```python
from build123d import *

# Parameters (mm, degrees)
SKETCH1_W           = 200
SKETCH1_H           = 200.3
BOSS_EXTRUDE1_DEPTH = 18
FILLET1_R           = 10
SKETCH2_W           = 150
SKETCH2_H           = 100
CUT_EXTRUDE1_DEPTH  = 13
FILLET2_R           = 10
SKETCH3_R           = 5
CUT_EXTRUDE2_DEPTH  = 5
SKETCH4_R           = 2.5
CUT_EXTRUDE3_DEPTH  = 143.123265161
SKETCH5_R           = 10
CUT_EXTRUDE4_DEPTH  = 143.123265161
SKETCH6_R           = 1.5
SKETCH6_W           = 23
SKETCH6_H           = 10
CUT_EXTRUDE5_DEPTH  = 143.667524335
FILLET3_R           = 3


with BuildPart() as part:
    # Sketch1 → Boss-Extrude1 (new body)
    with BuildSketch(Plane(origin=(0, 0, 0), x_dir=(1, 0, 0), z_dir=(0, 1, 0))):
        Rectangle(SKETCH1_W, SKETCH1_H)
    extrude(amount=BOSS_EXTRUDE1_DEPTH)

    # Fillet1
    fillet1_edges = [part.edges().sort_by_distance(p)[0] for p in [
        (100, 9, 100.15),
        (-100, 9, 100.15),
        (-100, 9, -100.15),
        (100, 9, -100.15),
    ]]
    fillet(fillet1_edges, radius=FILLET1_R)

    # Sketch2 → Cut-Extrude1 (cut)
    with BuildSketch(Plane.XZ):
        Rectangle(SKETCH2_W, SKETCH2_H)
    extrude(amount=-CUT_EXTRUDE1_DEPTH, mode=Mode.SUBTRACT)

    # Fillet2
    fillet2_edges = [part.edges().sort_by_distance(p)[0] for p in [
        (75, 6.5, 50),
        (75, 6.5, -50),
        (-75, 6.5, -50),
        (-75, 6.5, 50),
    ]]
    fillet(fillet2_edges, radius=FILLET2_R)

    # Sketch3 → Cut-Extrude2 (cut)
    with BuildSketch(Plane.XZ):
        with Locations(Location((-90, 90.15, 0), (0, 0, 270))):
            Circle(SKETCH3_R)
        with Locations(Location((90, 90.15, 0), (0, 0, 270))):
            Circle(SKETCH3_R)
        with Locations(Location((90, -90.15, 0), (0, 0, 270))):
            Circle(SKETCH3_R)
        with Locations(Location((-90, -90.15, 0), (0, 0, 270))):
            Circle(SKETCH3_R)
    extrude(amount=-CUT_EXTRUDE2_DEPTH, mode=Mode.SUBTRACT)

    # Sketch4 → Cut-Extrude3 (cut, through all)
    with BuildSketch(Plane.XZ.offset(-5)):
        with Locations(Location((-90, 90.15, 0), (0, 0, 270))):
            Circle(SKETCH4_R)
        with Locations(Location((90, 90.15, 0), (0, 0, 270))):
            Circle(SKETCH4_R)
        with Locations(Location((90, -90.15, 0), (0, 0, 270))):
            Circle(SKETCH4_R)
        with Locations(Location((-90, -90.15, 0), (0, 0, 270))):
            Circle(SKETCH4_R)
    extrude(amount=-CUT_EXTRUDE3_DEPTH, mode=Mode.SUBTRACT)

    # Sketch5 → Cut-Extrude4 (cut, through all)
    with BuildSketch(Plane.XZ.offset(-13)):
        with Locations(Location((0, 0, 0), (0, 0, 270))):
            Circle(SKETCH5_R)
    extrude(amount=-CUT_EXTRUDE4_DEPTH, mode=Mode.SUBTRACT)

    # Sketch6 → Cut-Extrude5 (cut, through all)
    with BuildSketch(Plane(origin=(0, 18, 0), x_dir=(1, 0, 0), z_dir=(0, 1, 0))):
        with Locations(Location((-28, -28, 0), (0, 0, 270))):
            Circle(SKETCH6_R)
        with Locations(Location((42, -20, 0), (0, 0, 270))):
            Circle(SKETCH6_R)
        with Locations(Location((-28, 28, 0), (0, 0, 90))):
            Circle(SKETCH6_R)
        with Locations(Location((42, 20, 0), (0, 0, 90))):
            Circle(SKETCH6_R)
        with Locations((0, -27)):
            Rectangle(SKETCH6_W, SKETCH6_H)
    extrude(amount=-CUT_EXTRUDE5_DEPTH, mode=Mode.SUBTRACT)

    # Fillet3
    fillet3_edges = [part.edges().sort_by_distance(p)[0] for p in [
        (11.5, 15.5, 22),
        (11.5, 15.5, 32),
        (-11.5, 15.5, 32),
        (-11.5, 15.5, 22),
    ]]
    fillet(fillet3_edges, radius=FILLET3_R)


solid = part.part
```
Read the model definition and answer for the solid it produces. Units are mm, in the model's axes. A direction names the side the tool comes from. Give positions to 0.01 mm unless a question says otherwise; leave off trailing zeros. Loops run counter-clockwise (first coordinate to the right, second up) from the corner with the lowest first, then second, coordinate; pieces in that order, holes last.
Item 1: For faces 1 (the cylindrical face through (-72.15, 6.59, -46.99)), 2 (the flat face through (0, 16, 22)), 3 (the cylindrical face through (-97.15, 9.13, 97.14)), determine the directions among +Z, -Z, +X, -X, +Y, -Y from which every point of the face is accessible in a straight line to the end or side of a thin tool.
Item 2: The part is cut by section B-B (x = 54.5). Write down the section's boundary in (y, z).
Item 3: The part is cut by section A-A (x = 0). Write down the section's boundary in (y, z).
Item 4: Each of these flat-tipped pins is pushed along its axis until it touches: pin 1 Ø2.5 at (x, z) = (-28, 28) entering from +Y; pin 2 Ø8 at (x, z) = (90.5, 90.5) entering from -Y. Where does it stop, or does it pass through?
Item 5: The mould has two halves that part along X. Classify faces 4 (the flat face through (-92, 5, 88)), 5 (the flat face through (-1, 18, 21)), 6 (the flat face through (100, 9, 1)): released by +X, released by -X, zero draft, split by the parting line, or undercut.
Item 6: Find the intervals of material crossed by line 1 along Z through (x, y) = (-43.5, 4); line 2 along X through (y, z) = (16.7, 28); line 3 along X through (y, z) = (2.15, 90.15), in increasing order.
Item 7: The part is cut by section C-C (x = -72.5). Write down the section's boundary in (y, z).
Taken from the geometry:
1. face 1: -Y
1. face 2: +Y, -Y
1. face 3: +Z, -X, +Y, -Y
2. outline: (0, -100.15) - (18, -100.15) - (18, 100.15) - (0, 100.15) - (0, 50) - (13, 50) - (13, -50) - (0, -50) - close
3. outline: (0, -100.15) - (18, -100.15) - (18, -10) - (13, -10) - (13, -50) - (0, -50) - close; (0, 50) - (13, 50) - (13, 32) - (18, 32) - (18, 100.15) - (0, 100.15) - close; (13, 10) - (18, 10) - (18, 22) - (13, 22) - close
4. pin 1: passes through
4. pin 2: stops at y = 5
5. face 4: undercut
5. face 5: zero draft
5. face 6: released by +X
6. line 1: z = -100.15 to -50, 50 to 100.15
6. line 2: x = -100 to -29.5, -26.5 to -11.5, 11.5 to 100
6. line 3: x = -100 to -95, -85 to 85, 95 to 100
7. outline: (0, -100.15) - (18, -100.15) - (18, 100.15) - (0, 100.15) - (0, 46.61) - (13, 46.61) - (13, -46.61) - (0, -46.61) - close
